The listing builds one solid part. Answer for the finished solid, in the listing's coordinates (mm). Round coordinates to 2 decimals unless told otherwise and drop trailing zeros. Write each loop counter-clockwise with the first axis right and the second up, starting at its lowest first coordinate (ties: lowest second). Pieces come first, ordered by that corner, then holes.
(1) A cutting plane is placed at B-B, the plane y = 1. Give the number of separate pieces and of enclosed holes in the cut face, and give its area (3 significant figures).
(2) The mould has two halves that part along Z. Classify faces 1 (the face through (18.38, 3.13, -26.64)), 2 (the face through (0, 3, -33.227)), 3 (the face through (0, 3, 6.773)): +Z half, -Z half, draft (parallel to the pull), parting line (faces both ways), or undercut.
(3) A cutting plane is placed at C-C, the plane x = 19. Give the vertices of the cut face in (y, z), and give its area (3 significant figures).
(4) A cutting plane is placed at D-D, the plane z = -22. Give the vertices of the cut face in (x, y), and give its area (3 significant figures).
(5) Find the intervals of material crossed by probe 1 along X at (y, z) = (0.75, -19.5); probe 2 along X at (y, z) = (1.5, -21); probe 3 along X at (y, z) = (3.75, -30), in increasing order.
(6) A cutting plane is placed at A-A, the plane x = 0. Give the vertices of the cut face in (y, z).
from build123d import *

# Parameters (mm, degrees)
CROQUIS1_W              = 50.8
CROQUIS1_H              = 80
SALIENTE_EXTRUIR1_DEPTH = 6.35
CROQUIS4_R              = 4
CORTAR_EXTRUIR3_DEPTH   = 48.806720239
CROQUIS5_W              = 50.8
CROQUIS5_H              = 12.7
CORTAR_EXTRUIR4_DEPTH   = 48.806720239
CROQUIS6_W              = 50.8
CROQUIS6_H              = 20.526572449
CORTAR_EXTRUIR5_DEPTH   = 10
CROQUIS7_W              = 50.8
CROQUIS7_H              = 6.773427551
CORTAR_EXTRUIR6_DEPTH   = 10
CROQUIS9_R              = 5
CORTAR_EXTRUIR7_DEPTH   = 10
CROQUIS10_R             = 2
CORTAR_EXTRUIR8_DEPTH   = 10


with BuildPart() as part:
    # Croquis1 → Saliente-Extruir1 (new body)
    with BuildSketch(Plane(origin=(0, 0, 0), x_dir=(1, 0, 0), z_dir=(0, 1, 0))):
        Rectangle(CROQUIS1_W, CROQUIS1_H)
    extrude(amount=SALIENTE_EXTRUIR1_DEPTH)

    # Croquis4 → Cortar-Extruir3 (cut, through all)
    with BuildSketch(Plane(origin=(0, 6.35, 0), x_dir=(1, 0, 0), z_dir=(0, 1, 0))):
        with Locations(Location((-19, 19.466091849, 0), (0, 0, 270))):
            Circle(CROQUIS4_R)
        with Locations(Location((19, 19.466091849, 0), (0, 0, 270))):
            Circle(CROQUIS4_R)
        with Locations(Location((0, 0.466091849, 0), (0, 0, 270))):
            Circle(CROQUIS4_R)
    extrude(amount=-CORTAR_EXTRUIR3_DEPTH, mode=Mode.SUBTRACT)

    # Croquis5 → Cortar-Extruir4 (cut, through all)
    with BuildSketch(Plane(origin=(0, 6.35, 0), x_dir=(1, 0, 0), z_dir=(0, 1, 0))):
        with Locations((0, -33.65)):
            Rectangle(CROQUIS5_W, CROQUIS5_H)
    extrude(amount=-CORTAR_EXTRUIR4_DEPTH, mode=Mode.SUBTRACT)

    # Croquis6 → Cortar-Extruir5 (cut)
    with BuildSketch(Plane(origin=(0, 6.35, 0), x_dir=(1, 0, 0), z_dir=(0, 1, 0))):
        with Locations((0, -17.036713776)):
            Rectangle(CROQUIS6_W, CROQUIS6_H)
    extrude(amount=-CORTAR_EXTRUIR5_DEPTH, mode=Mode.SUBTRACT)

    # Croquis7 → Cortar-Extruir6 (cut)
    with BuildSketch(Plane.XZ):
        with Locations((0, -36.613286225)):
            Rectangle(CROQUIS7_W, CROQUIS7_H)
    extrude(amount=-CORTAR_EXTRUIR6_DEPTH, mode=Mode.SUBTRACT)

    # Croquis9 → Cortar-Extruir7 (cut)
    with BuildSketch(Plane.XZ):
        with Locations(Location((0, -19.466091849, 0), (0, 0, 270))):
            Circle(CROQUIS9_R)
    extrude(amount=-CORTAR_EXTRUIR7_DEPTH, mode=Mode.SUBTRACT)

    # Croquis10 → Cortar-Extruir8 (cut)
    with BuildSketch(Plane.XZ):
        with Locations(Location((-20.4, 1.773427551, 0), (0, 0, 270))):
            Circle(CROQUIS10_R)
        with Locations(Location((19.6, 1.773427551, 0), (0, 0, 270))):
            Circle(CROQUIS10_R)
        with Locations(Location((19.6, -28.226572449, 0), (0, 0, 270))):
            Circle(CROQUIS10_R)
        with Locations(Location((-20.4, -28.226572449, 0), (0, 0, 270))):
            Circle(CROQUIS10_R)
    extrude(amount=-CORTAR_EXTRUIR8_DEPTH, mode=Mode.SUBTRACT)


solid = part.part
Solutions:
1. separate pieces: 1
1. enclosed holes: 8
1. area: 1,750 mm2
2. face 1: undercut
2. face 2: -Z half
2. face 3: +Z half
3. outline: (0, -33.23) - (6.35, -33.23) - (6.35, -30.13) - (0, -30.13) - close; (0, -26.32) - (6.35, -26.32) - (6.35, -23.47) - (0, -23.47) - close; (0, -15.47) - (6.35, -15.47) - (6.35, -0.13) - (0, -0.13) - close; (0, 3.68) - (6.35, 3.68) - (6.35, 6.77) - (0, 6.77) - close
3. area: 155 mm2
4. outline: (-25.4, 0) - (-22.1, 0) - (-22.1, 6.35) - (-25.4, 6.35) - close; (-15.9, 0) - (-4.31, 0) - (-4.31, 6.35) - (-15.9, 6.35) - close; (4.31, 0) - (15.9, 0) - (15.9, 6.35) - (4.31, 6.35) - close; (22.1, 0) - (25.4, 0) - (25.4, 6.35) - (22.1, 6.35) - close
4. area: 189 mm2
5. probe 1: x = -25.4 to -23, -15 to -5, 5 to 15, 23 to 25.4
5. probe 2: x = -25.4 to -22.69, -15.31 to -4.76, 4.76 to 15.31, 22.69 to 25.4
5. probe 3: x = -25.4 to -21.32, -19.48 to 18.68, 20.52 to 25.4
6. outline: (0, -33.23) - (6.35, -33.23) - (6.35, -24.47) - (0, -24.47) - close; (0, -14.47) - (6.35, -14.47) - (6.35, -4.47) - (0, -4.47) - close; (0, 3.53) - (6.35, 3.53) - (6.35, 6.77) - (0, 6.77) - close
